```python
from build123d import *

# Parameters (mm, degrees)
F0_W           = 174.0000014603
F0_H           = 43.0000014603
F1_DEPTH       = 6
F0_W_2         = 17
F0_H_2         = 25
F0_R           = 3
F2_DEPTH       = 4
F3_W           = 12
F3_H           = 18
F4_DEPTH       = 6
F5_D           = 5.5
F5_CBORE_D     = 9.75
F5_CBORE_DEPTH = 5
F6_SIZE        = 2
F7_R           = 3
F8_R           = 1.5


with BuildPart() as f1:
    # F0 (on Top) → F1 (new body)
    with BuildSketch(Plane.XY):
        Polygon((93, -12.5), (93, 12.5), (93, 27.5), (-93, 27.5), (-93, 12.5), (-93, -12.5), (-93, -27.5), (93, -27.5), align=None)
        Rectangle(F0_W, F0_H, mode=Mode.SUBTRACT)
    extrude(amount=F1_DEPTH)

    # F0 (on Top) → F2 (join)
    with BuildSketch(Plane.XY):
        with Locations((101.5, 0)):
            Rectangle(F0_W_2, F0_H_2)
        with Locations((100, 0)):
            Circle(F0_R, mode=Mode.SUBTRACT)
        Polygon((93, -12.5), (93, 12.5), (93, 27.5), (-93, 27.5), (-93, 12.5), (-93, -12.5), (-93, -27.5), (93, -27.5), align=None)
        Rectangle(F0_W, F0_H, mode=Mode.SUBTRACT)
        with Locations((-101.5, 0)):
            Rectangle(F0_W_2, F0_H_2)
        with Locations((-100, 0)):
            Circle(F0_R, mode=Mode.SUBTRACT)
    extrude(amount=F2_DEPTH)

    # F3 (on face) → F4 (join)
    with BuildSketch(Plane.XY.offset(6)):
        with Locations((-50, 12.5000007302)):
            Rectangle(F3_W, F3_H)
        with Locations((50, 12.5000007302)):
            Rectangle(F3_W, F3_H)
    extrude(amount=-F4_DEPTH)

    # F5 (through all)
    with Locations(Plane(origin=(0, 0, 0), x_dir=(1, 0, 0), z_dir=(0, 0, -1))):
        with Locations((-50, -10.8), (50, -10.8)):
            CounterBoreHole(F5_D / 2, F5_CBORE_D / 2, F5_CBORE_DEPTH)

    # F6
    f6_edges = [f1.edges().sort_by_distance(p)[0] for p in [
        (97, 0, 4),
        (-103, 0, 4),
    ]]
    chamfer(f6_edges, length=F6_SIZE)

    # F7
    f7_edges = [f1.edges().sort_by_distance(p)[0] for p in [
        (-110, 0, 4),
        (-101.5, 12.5, 4),
        (-101.5, -12.5, 4),
        (101.5, 12.5, 4),
        (110, 0, 4),
        (101.5, -12.5, 4),
    ]]
    fillet(f7_edges, radius=F7_R)

    # F8
    f8_edges = [f1.edges().sort_by_distance(p)[0] for p in [
        (0, 27.5, 6),
        (-93, 0, 6),
        (0, -27.5, 6),
        (93, 0, 6),
    ]]
    fillet(f8_edges, radius=F8_R)


solid = f1.part
```
For this review, take the finished solid that the model builds, in its own axes (mm). A direction names the side the tool comes from. Coordinates: 2 decimals unless noted, no trailing zeros. Write each loop counter-clockwise with the first axis right and the second up, starting at its lowest first coordinate (ties: lowest second). Pieces come first, ordered by that corner, then holes.
(1) Add section A-A on x = 100. Give the boundary of the cut face in (y, z).
(2) Add section D-D on x = 62. Give the boundary of the cut face in (y, z).
(3) Wall thickness on probe 1 along X at (y, z) = (20, 0.9); probe 2 along X at (y, z) = (10.5, 0.3); probe 3 along X at (y, z) = (-4, 0.5): over which ranges is each line inside the solid? List them lowest first.
(4) For pin 1 Ø0.8 at (x, z) = (-100, 0.5) entering from -Y; pin 2 Ø5 at (x, y) = (51.5, 10) entering from -Z; pin 3 Ø3 at (y, z) = (5, 4.5) entering from -X; pin 4 Ø5 at (x, y) = (100, 0) entering from -Z, all flat-tipped, find the tip position at first contact; note any pin that passes through.
(5) Tool access review of faces 4 (the face through (52, 13, 5)), 5 (the face through (-1, -21.5, 3)), 6 (the face through (1, 27.5, 2)): name each direction out of +Z, -Z, +X, -X, +Y, -Y from which nothing blocks a thin tool from reaching the whole face with its end or side.
(6) Add section B-B on y = 0. Give the boundary of the cut face in (x, z), then the cut area to 3 significant figures.
(7) The part is to be moulded in two halves that separate along X. For faces 1 (the face through (-48, 13, 5)), 2 (the face through (95, 2, 4)), 3 (the face through (93, -0.4, 4.2)), say which applies: +X half, -X half, draft (parallel to the pull), parting line (faces both ways), or undercut.
(8) Add section C-C on x = -50. Give the boundary of the cut face in (y, z) (3 decimals).
Answer sheet:
1. outline: (-12.5, 0) - (-3, 0) - (-3, 2) - (-5, 4) - (-9.5, 4) arc R3 ccw to (-12.5, 1) - close; (3, 0) - (12.5, 0) - (12.5, 1) arc R3 ccw to (9.5, 4) - (5, 4) - (3, 2) - close
2. outline: (-27.5, 0) - (-21.5, 0) - (-21.5, 6) - (-26, 6) arc R1.5 ccw to (-27.5, 4.5) - close; (21.5, 0) - (27.5, 0) - (27.5, 4.5) arc R1.5 ccw to (26, 6) - (21.5, 6) - close
3. probe 1: x = -93 to -87, -56 to -44, 44 to 56, 87 to 93
3. probe 2: x = -110 to -87, -56 to -54.87, -45.13 to -44, 44 to 45.13, 54.87 to 56, 87 to 110
3. probe 3: x = -110 to -87, 87 to 110
4. pin 1: stops at y = -12.5
4. pin 2: stops at z = 5
4. pin 3: stops at x = -109.24
4. pin 4: passes through
5. face 4: -Z
5. face 5: +Z, -Z
5. face 6: +Z, -Z, +X, -X, +Y
6. outline: (-110, 0) - (-103, 0) - (-103, 2) - (-105, 4) - (-107, 4) arc R3 ccw to (-110, 1) - close; (-97, 0) - (-87, 0) - (-87, 6) - (-91.5, 6) arc R1.5 ccw to (-93, 4.5) - (-93, 4) - (-95, 4) - (-97, 2) - close; (87, 0) - (97, 0) - (97, 2) - (95, 4) - (93, 4) - (93, 4.5) arc R1.5 ccw to (91.5, 6) - (87, 6) - close; (103, 0) - (110, 0) - (110, 1) arc R3 ccw to (107, 4) - (105, 4) - (103, 2) - close
6. area: 147 mm2
7. face 1: undercut
7. face 2: draft
7. face 3: +X half
8. outline: (-27.5, 0) - (-21.5, 0) - (-21.5, 6) - (-26, 6) arc R1.5 ccw to (-27.5, 4.5) - close; (3.5, 0) - (5.925, 0) - (5.925, 5) - (8.05, 5) - (8.05, 6) - (3.5, 6) - close; (13.55, 5) - (15.675, 5) - (15.675, 0) - (27.5, 0) - (27.5, 4.5) arc R1.5 ccw to (26, 6) - (13.55, 6) - close
